Study the drawing (mm; zero at the part's minimum x, y, z) and answer. A direction names the side the tool comes from. Coordinates: 2 decimals unless noted, no trailing zeros. Order: outer loops, then holes, each group sorted by start corner. A loop starts at its lowest first (then second) coordinate and runs counter-clockwise, first axis right, second up. Notation, with made-up numbers: M 49,41 L 98,41 A27 ccw 98,73 Z; hole C 53,-24 d6. An arc over 180 degrees is marked long. Put each result on its own line as item: value.
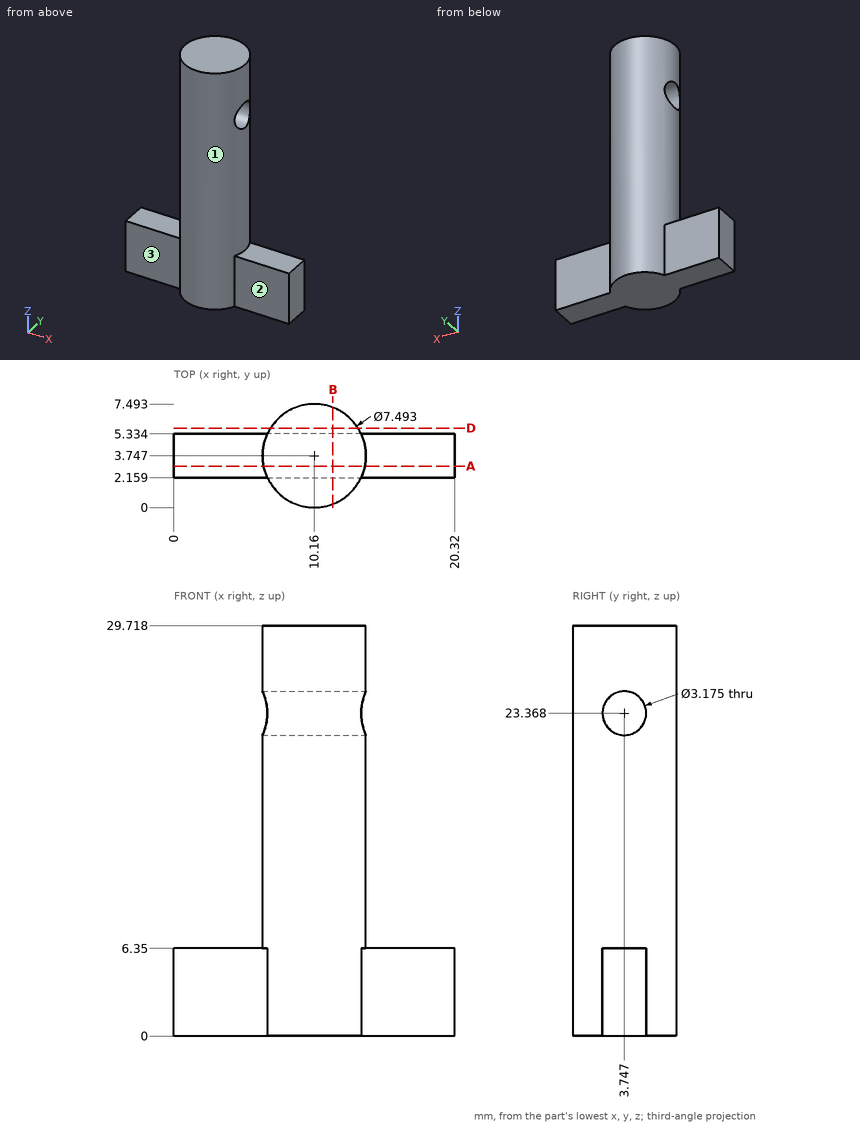
Q1. A tool of negligible diameter and unlimited length cuts with its end or side. For the marked faces 1, 2 and 3, from which of +Z, -Z, +X, -X, +Y, -Y can it reach the whole face along a straight path? Write none if from no direction.
Answers below:
face 1: +Z
face 2: +Z, -Z, +X, -Y
face 3: +Z, -Z, -X, -Y
Q2. Find section B-B on x = 11.5. Write down the section's boundary in (y, z) (1 decimal), plus the area to 3 significant figures.
Answers below:
outline: M 0.2,0 L 7.2,0 L 7.2,29.7 L 0.2,29.7 Z; hole C 3.7,23.4 d3.2
area: 200 mm^2
Q3. Consider line 1 along Y through (x, z) = (5.25, 5) (1 decimal); line 2 along Z through (x, y) = (17.5, 5); line 3 along X through (y, z) = (3.75, 28.5). Determine where each line is inside the solid, lowest interval first.
Answers below:
line 1: y = 2.2 to 5.3
line 2: z = 0 to 6.35
line 3: x = 6.41 to 13.91
Q4. Find section D-D on y = 5.75. Write down the section's boundary in (x, z) (1 decimal), plus the area to 3 significant figures.
Answers below:
outline: M 7,0 L 13.3,0 L 13.3,29.7 L 7,29.7 Z
area: 188 mm^2
Q5. Given pin 1 (8 mm diameter, centred on x = 5, z = 11.5, fed in from -Y) (1 decimal); pin 2 (1.5 mm diameter, centred on y = 3.5, z = 23, fed in from +X); pin 3 (1.9 mm diameter, centred on x = 16.5, z = 2.5, fed in from -Y); pin 4 (1.9 mm diameter, centred on x = 16.5, z = 3.5, fed in from +Y), each flat-ended and moving along its own axis, determine where each tip first touches the part or whether it passes through.
Answers below:
pin 1: stops at y = 0.2
pin 2: passes through
pin 3: stops at y = 2.16
pin 4: stops at y = 5.33
Q6. Find section A-A on y = 3. Write down the section's boundary in (x, z), plus the area to 3 significant figures.
Answers below:
outline: M 0,0 L 20.32,0 L 20.32,6.35 L 13.83,6.35 L 13.83,21.97 L 6.49,21.97 L 6.49,6.35 L 0,6.35 Z; M 6.49,24.77 L 13.83,24.77 L 13.83,29.72 L 6.49,29.72 Z
area: 280 mm^2
